from build123d import *

# Parameters (mm, degrees)
F0_R      = 3
F1_DEPTH  = 7
F2_R      = 11.15
F3_DEPTH  = 26.25
F4_R      = 8
F5_DEPTH  = 6.85
F6_R      = 6
F7_DEPTH  = 5.88
F8_R      = 8
F9_DEPTH  = 4
F11_DEPTH = 8.8
F12_R     = 3.75
F13_DEPTH = 0.75
F14_R     = 5
F15_DEPTH = 2.5


with BuildPart() as f1:
    # F0 (on Top) → F1 (new body)
    with BuildSketch(Plane.XY):
        Circle(F0_R)
    extrude(amount=F1_DEPTH)

    # F2 (on face) → F3 (join)
    with BuildSketch(Plane.XY.offset(7)):
        Circle(F2_R)
    extrude(amount=F3_DEPTH)

    # F4 (on face) → F5 (join)
    with BuildSketch(Plane.XY.offset(33.25)):
        Circle(F4_R)
    extrude(amount=F5_DEPTH)

    # F6 (on face) → F7 (join)
    with BuildSketch(Plane.XY.offset(40.1)):
        Circle(F6_R)
    extrude(amount=F7_DEPTH)

    # F8 (on face) → F9 (join)
    with BuildSketch(Plane.XY.offset(45.98)):
        Circle(F8_R)
    extrude(amount=F9_DEPTH)

    # F10 (on face) → F11 (join)
    with BuildSketch(Plane.XY.offset(49.98)):
        Polygon((-4.95, 2.8578838325), (-4.95, -2.8578838325), (0, -5.715767665), (4.95, -2.8578838325), (4.95, 2.8578838325), (0, 5.715767665), align=None)
    extrude(amount=F11_DEPTH)

    # F12 (on face) → F13 (join)
    with BuildSketch(Plane.XY.offset(58.78)):
        Circle(F12_R)
    extrude(amount=F13_DEPTH)

    # F14 (on face) → F15 (join)
    with BuildSketch(Plane.XY.offset(59.53)):
        Circle(F14_R)
    extrude(amount=F15_DEPTH)


solid = f1.part
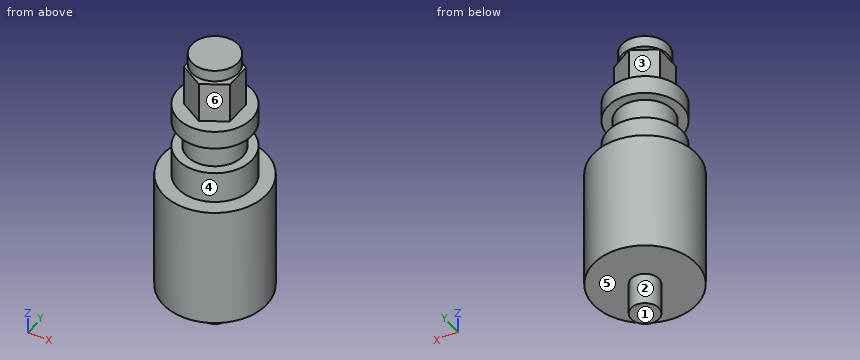
The model under review builds one solid part; all positions refer to its coordinate system, in mm. Face numbers are marked on the shaded views. A direction names the side the tool comes from. Round coordinates to 2 decimals unless told otherwise and drop trailing zeros. Loops run counter-clockwise (first coordinate to the right, second up) from the corner with the lowest first, then second, coordinate; pieces in that order, holes last. Notation, with made-up numbers: (-6.5, -22.5) -> (35.5, -22.5) arc R15 ccw to (35.5, 0.5) -> close; hole circle Ø3 at (-29, 13.5). An arc over 180 degrees is marked (long way). Return JSON: item names as keys, results as strings.
(1) For the marked faces 4, 5 and 6, list the 3-axis set-ups (+Z, -Z, +X, -X, +Y, -Y) from which the entire face can be reached by the end or side of a thin tool; tool diameter is ignored.
Solved:
{"face 4": "+Z", "face 5": "-Z", "face 6": "+X, -Y"}
(2) Add section D-D on z = 56.5. Write out the cut boundary in (x, y), plus the area to 3 significant figures.
Solved:
{"outline": "(-4.95, -2.86) -> (0, -5.72) -> (4.95, -2.86) -> (4.95, 2.86) -> (0, 5.72) -> (-4.95, 2.86) -> close", "area": "84.9 mm2"}
(3) The part is to be moulded in two halves that separate along Z. For the marked faces 1, 2 and 3, say which applies: released by +Z, released by -Z, zero draft, split by the parting line, or undercut.
Solved:
{"face 1": "released by -Z", "face 2": "zero draft", "face 3": "undercut"}
(4) For line 1 (Z direction, x = 1.75, y = 6.25); line 2 (Z direction, x = 8.5, y = 7); line 3 (Z direction, x = 1.5, y = 3), list the stretches that pass through material, from the lowest coordinate up.
Solved:
{"line 1": "7 to 40.1, 45.98 to 49.98", "line 2": "7 to 33.25", "line 3": "7 to 62.03"}
(5) Add section A-A on y = -6.75. Write out the cut boundary in (x, z), plus the area to 3 significant figures.
Solved:
{"outline": "(-8.87, 7) -> (8.87, 7) -> (8.87, 33.25) -> (4.29, 33.25) -> (4.29, 40.1) -> (-4.29, 40.1) -> (-4.29, 33.25) -> (-8.87, 33.25) -> close; (-4.29, 45.98) -> (4.29, 45.98) -> (4.29, 49.98) -> (-4.29, 49.98) -> close", "area": "559 mm2"}
(6) Add section C-C on z = 12. Write out the cut boundary in (x, y).
Solved:
{"outline": "circle Ø22.3 at (0, 0)"}
(7) For pin 1 (4.5 mm diameter, centred on y = -0.5, z = 53.5, fed in from -X); pin 2 (1 mm diameter, centred on x = -8.5, z = 32.5, fed in from -Y); pin 3 (3 mm diameter, centred on x = 0, z = 43, fed in from +Y); pin 4 (5 mm diameter, centred on x = -9, z = 55, fed in from -Y), all flat-tipped, find the tip position at first contact; note any pin that passes through.
Solved:
{"pin 1": "x = -4.95", "pin 2": "y = -7.77", "pin 3": "y = 6", "pin 4": "through"}
